The listing builds one solid part. Answer for the finished solid, in the listing's coordinates (mm). A direction names the side the tool comes from. Round coordinates to 2 decimals unless told otherwise and drop trailing zeros. Order: outer loops, then holes, each group sorted by start corner. A loop starts at its lowest first (then second) coordinate and runs counter-clockwise, first axis right, second up. Notation, with made-up numbers: (48, 18.5) - (64, 18.5) arc R12 cw to (64, 28.5) - close; hole circle Ø11 at (-10.5, 37). An arc over 180 degrees is marked (long way). Write item = value, one per line.
Autodesk Inventor part; units mm, degrees
ref_plane "YZ Plane" through (0, 0, 0) normal (1, 0, 0) x (0, 1, 0)
ref_plane "XZ Plane" through (0, 0, 0) normal (0, 1, 0) x (-1, 0, 0)
ref_plane "XY Plane" through (0, 0, 0) normal (0, 0, 1) x (1, 0, 0)
sketch "Sketch2" plane through (0, 0, 0) normal (0, 0, 1) x (1, 0, 0)
  line L0 (-17, 28) -> (0, 28)
  line L1 (0, 28) -> (0, 17)
  line L2 (0, 17) -> (4, 17)
  line L3 (4, 17) -> (4, 7)
  line L4 (4, 7) -> (0, 7)
  line L5 (0, 7) -> (0, 0)
  line L6 (0, 0) -> (-17, 0)
  line L7 (-17, 0) -> (-17, 7)
  line L8 (-17, 7) -> (-21, 7)
  line L9 (-21, 7) -> (-21, 17)
  line L10 (-21, 17) -> (-17, 17)
  line L11 (-17, 28) -> (-17, 17)
  dimension "d0" = 17
  dimension "d1" = 28
  dimension "d2" = 4
  dimension "d3" = 7
  dimension "d4" = 10
extrude "Extrusion1" add sketch "Sketch2" along normal blind 5
sketch "Sketch4" plane through (0, 0, 0) normal (0, 0, -1) x (-1, 0, 0)
  line L0 (17, 28) -> (0, 28)
  line L1 (0, 28) -> (0, 17)
  line L2 (0, 17) -> (-4, 17)
  line L3 (-4, 17) -> (-4, 7)
  line L4 (-4, 7) -> (0, 7)
  line L5 (0, 7) -> (0, 0)
  line L6 (0, 0) -> (17, 0)
  line L7 (17, 0) -> (17, 7)
  line L8 (17, 7) -> (21, 7)
  line L9 (21, 7) -> (21, 17)
  line L10 (21, 17) -> (17, 17)
  line L11 (17, 17) -> (17, 28)
  line L12 (0, 28) -> (17, 28)
  line L13 (11.5, 24) -> (11.5, 4)
  line L14 (11.5, 4) -> (5.5, 4)
  line L15 (5.5, 4) -> (5.5, 24)
  line L16 (5.5, 24) -> (11.5, 24)
  dimension "d15" = 6
  dimension "d17" = 5.5
  dimension "d30" = 20
  dimension "d31" = 4
extrude "Extrusion3" cut sketch "Sketch4" against normal blind 1.5 contours L13 L14 L15 L16
sketch "Sketch5" plane through (0, 0, 5) normal (0, 0, 1) x (1, 0, 0)
  line L0 (0, 28) -> (-17, 28)
  line L1 (-17, 28) -> (-17, 17)
  line L2 (-17, 17) -> (-21, 17)
  line L3 (-21, 17) -> (-21, 7)
  line L4 (-21, 7) -> (-17, 7)
  line L5 (-17, 7) -> (-17, 0)
  line L6 (-17, 0) -> (0, 0)
  line L7 (0, 0) -> (0, 7)
  line L8 (0, 7) -> (4, 7)
  line L9 (4, 7) -> (4, 17)
  line L10 (4, 17) -> (0, 17)
  line L11 (0, 17) -> (0, 28)
  line L12 (-21, 17) -> (4, 7)
  line L13 (-21.4753, 7) -> (4, 17)
  circle A0 centre (-8.6177, 12.0471) radius 5
  dimension "d20" = 10
  dimension "d21" = 12.0471
extrude "Extrusion4" cut sketch "Sketch5" against normal through all contours A0 L12 L13 | L13 L12 A0 | L12 L13 A0 | A0 L13 L12
sketch "Sketch6" plane through (0, 0, 5) normal (0, 0, 1) x (1, 0, 0)
  circle A0 centre (-8.6177, 12.0471) radius 5
  line L0 (0, 28) -> (-17, 28)
  line L1 (-17, 28) -> (-17, 17)
  line L2 (-17, 17) -> (-21, 17)
  line L3 (-21, 17) -> (-21, 7)
  line L4 (-21, 7) -> (-17, 7)
  line L5 (-17, 7) -> (-17, 0)
  line L6 (-17, 0) -> (0, 0)
  line L7 (0, 0) -> (0, 7)
  line L8 (0, 7) -> (4, 7)
  line L9 (4, 7) -> (4, 17)
  line L10 (4, 17) -> (0, 17)
  line L11 (0, 17) -> (0, 28)
  circle A1 centre (-12.5, 26) radius 1.35
  dimension "d24" = 2.7
  dimension "d25" = 4.5
  dimension "d26" = 2
extrude "Extrusion5" cut sketch "Sketch6" against normal through all contours A1
sketch "Sketch7" plane through (0, 0, 5) normal (0, 0, 1) x (1, 0, 0)
  line L0 (0, 0) -> (0, 7)
  line L1 (-17, 0) -> (0, 0)
  circle A0 centre (-4.5, 5) radius 1.35
  dimension "d32" = 2.7
  dimension "d33" = 4.5
  dimension "d34" = 5
extrude "Extrusion6" cut sketch "Sketch7" against normal through all
sketch "Sketch8" plane through (4, 7, 0) normal (1, 0, 0) x (0, 0, -1)
  line L0 (0, 10) -> (0, 0)
  line L1 (0, 10) -> (-5, 10)
  line L2 (-5, 0) -> (-5, 10)
  line L3 (0, 0) -> (-5, 0)
  circle A0 centre (-1.5, 5) radius 1.35
  point P0 (0, -7)
  dimension "d37" = 2.7
  dimension "d38" = 1.5
extrude "Extrusion7" cut sketch "Sketch8" against normal through all contours A0
properties part number "tapa"
Q1. Section B-B on z = 1 is taken. Count the separate pieces of the cut face and the enclosed holes in it, then the cut area to 3 significant figures.
Model answer:
separate_pieces = 2
enclosed_holes = 1
area = 365 mm^2
Q2. Flat-ended cylindrical pins translate along their axes: P1, Ø2, axis at x = 2, z = 3, coming from the -Y side; P2, Ø2.5, axis at y = 12, z = 1.5, coming from the -X side; P3, Ø0.8, axis at y = 21, z = 1, coming from the -X side; P4, Ø1.6, axis at y = 5.5, z = 1, coming from the +X side. Find the tip coordinate at first contact, or state that the pin passes through.
Model answer:
P1 = 7
P2 = through
P3 = -17
P4 = 0
Q3. Section C-C on y = 22.25 is taken. Determine the outline of the cut face in (x, z).
Model answer:
outline = (-17, 0) - (-11.5, 0) - (-11.5, 1.5) - (-5.5, 1.5) - (-5.5, 0) - (0, 0) - (0, 5) - (-17, 5) - close
Q4. Find the intervals of material crossed by line 1 (Y direction, x = -4.5, z = 3.55); line 2 (X direction, y = 5, z = 1.6); line 3 (Z direction, x = -1.5, y = 12), in increasing order. Write a range as from..to.
Model answer:
line_1 = 0..3.65, 6.35..9.21, 14.88..28
line_2 = -17..-5.85, -3.15..0
line_3 = 0..0.15, 2.85..5
Q5. For faces 1 (the face through (0, 4, 2)), 2 (the face through (-19, 7, 2)), 3 (the face through (-5.5, 7, 1)), 4 (the face through (-3.212, 5.406, 2.535)), determine the directions among +Z, -Z, +X, -X, +Y, -Y from which every point of the face is accessible in a straight line to the end or side of a thin tool.
Model answer:
face_1 = +Z, -Z, +X, -Y
face_2 = +Z, -Z, -X, -Y
face_3 = -Z
face_4 = +Z, -Z
Q6. Section D-D on z = 3.85 is taken. Determine the outline of the cut face in (x, y).
Model answer:
outline = (-21, 7) - (-17, 7) - (-17, 0) - (0, 0) - (0, 7) - (4, 7) - (4, 17) - (0, 17) - (0, 28) - (-17, 28) - (-17, 17) - (-21, 17) - close; hole circle Ø2.7 at (-12.5, 26); hole circle Ø10 at (-8.62, 12.05); hole circle Ø2.7 at (-4.5, 5)
Q7. Determine the mould class of faces 5 (the face through (0.146, 13.339, 1.676)), 6 (the face through (2, 17, 2)), 7 (the face through (-3, 14, 0)) for opening direction Z: released by +Z, released by -Z, zero draft, split by the parting line, or undercut.
Model answer:
face_5 = undercut
face_6 = zero draft
face_7 = released by -Z
Q8. Section A-A on y = 5 is taken. Determine the outline of the cut face in (x, z), then the cut area to 3 significant figures.
Model answer:
outline = (-17, 0) - (-11.5, 0) - (-11.5, 1.5) - (-5.85, 1.5) - (-5.85, 5) - (-17, 5) - close; (-3.15, 0) - (0, 0) - (0, 5) - (-3.15, 5) - close
area = 63.0 mm^2
